from build123d import *

# Parameters (mm, degrees)
F0_W     = 50.8
F0_H     = 50.8
F1_DEPTH = 50.8
F2_R     = 12.7
F3_DEPTH = 12.7
F4_R     = 12.7
F5_DEPTH = 50.8


with BuildPart() as f1:
    # F0 (on Front) → F1 (new body)
    with BuildSketch(Plane.XZ):
        with Locations((-6.564537, 3.794339)):
            Rectangle(F0_W, F0_H)
    extrude(amount=F1_DEPTH)

    # F2 (on face) → F3 (join)
    with BuildSketch(Plane.XZ.offset(50.8)):
        with Locations((-6.564537, 3.794339)):
            Circle(F2_R)
    extrude(amount=F3_DEPTH)

    # F4 (on face) → F5 (cut)
    with BuildSketch(Plane.XY.offset(29.194339)):
        with Locations((-6.564537, -25.4)):
            Circle(F4_R)
    extrude(amount=-F5_DEPTH, mode=Mode.SUBTRACT)


solid = f1.part
The model under review builds one solid part; all positions refer to its coordinate system, in mm. A direction names the side the tool comes from. Give positions to 0.01 mm unless a question says otherwise; leave off trailing zeros. Order: outer loops, then holes, each group sorted by start corner. A loop starts at its lowest first (then second) coordinate and runs counter-clockwise, first axis right, second up. Notation, with made-up numbers: (30, 18) -> (53, 18) arc R7 ccw to (53, 24) -> close; hole circle Ø3 at (31, -17.5). An arc over 180 degrees is marked (long way). Write item = value, one per line. Start each with the question number.
(1) For L1, parallel to Y at x = 7.5, z = -8.5; L2, parallel to Y at x = 1, z = 1.5; L3, parallel to Y at x = -3.5, z = -10.5, list the stretches that pass through material, from the lowest coordinate up. Write a range as from..to.
(2) Take a section at D-D (x = -24.5). Write out the cut boundary in (y, z), plus the area to 3 significant figures.
(3) For pin 1 Ø5 at (x, z) = (-25.5, 6) entering from -Y, flat-tipped, find the tip position at first contact; note if it passes through.
(4) Tool access review of faces 4 (the flat face through (-18, -19, -21.606)), 5 (the cylindrical face through (-16.643, -57.061, -3.933)): name each direction out of +Z, -Z, +X, -X, +Y, -Y from which nothing blocks a thin tool from reaching the whole face with its end or side.
(5) Take a section at C-C (x = -17.5). Write out the cut boundary in (y, z), plus the area to 3 significant figures.
(6) Take a section at A-A (y = -25.4). Write out the cut boundary in (x, z).
(7) Take a section at B-B (z = 24). Write out the cut boundary in (x, y).
(8) Draft analysis for pull direction X (two halves, no side actions). For faces 1 (the flat face through (18.835, -25, 3)), 2 (the flat face through (-13, -50.8, 15)), 3 (the cylindrical face through (-9.3, -37.8, 4.1)), state which applies: +X half, -X half, draft (parallel to the pull), parting line (faces both ways), or undercut.
Returned:
q1.L1 = -50.8..0
q1.L2 = -63.5..-35.6, -15.2..0
q1.L3 = -50.8..-37.72, -13.08..0
q2.outline = (-50.8, -21.61) -> (0, -21.61) -> (0, 29.19) -> (-50.8, 29.19) -> close
q2.area = 2,580 mm²
q3.pin_1 = -50.8
q4.face_4 = -Z, +X, -X, +Y, -Y
q4.face_5 = -Y
q5.outline = (-63.5, -2.66) -> (-50.8, -2.66) -> (-50.8, -21.61) -> (-31.86, -21.61) -> (-31.86, 29.19) -> (-50.8, 29.19) -> (-50.8, 10.25) -> (-63.5, 10.25) -> close; (-18.94, -21.61) -> (0, -21.61) -> (0, 29.19) -> (-18.94, 29.19) -> close
q5.area = 2,090 mm²
q6.outline = (-31.96, -21.61) -> (-19.26, -21.61) -> (-19.26, 29.19) -> (-31.96, 29.19) -> close; (6.14, -21.61) -> (18.84, -21.61) -> (18.84, 29.19) -> (6.14, 29.19) -> close
q7.outline = (-31.96, -50.8) -> (18.84, -50.8) -> (18.84, 0) -> (-31.96, 0) -> close; hole circle Ø25.4 at (-6.56, -25.4)
q8.face_1 = +X half
q8.face_2 = draft
q8.face_3 = undercut
